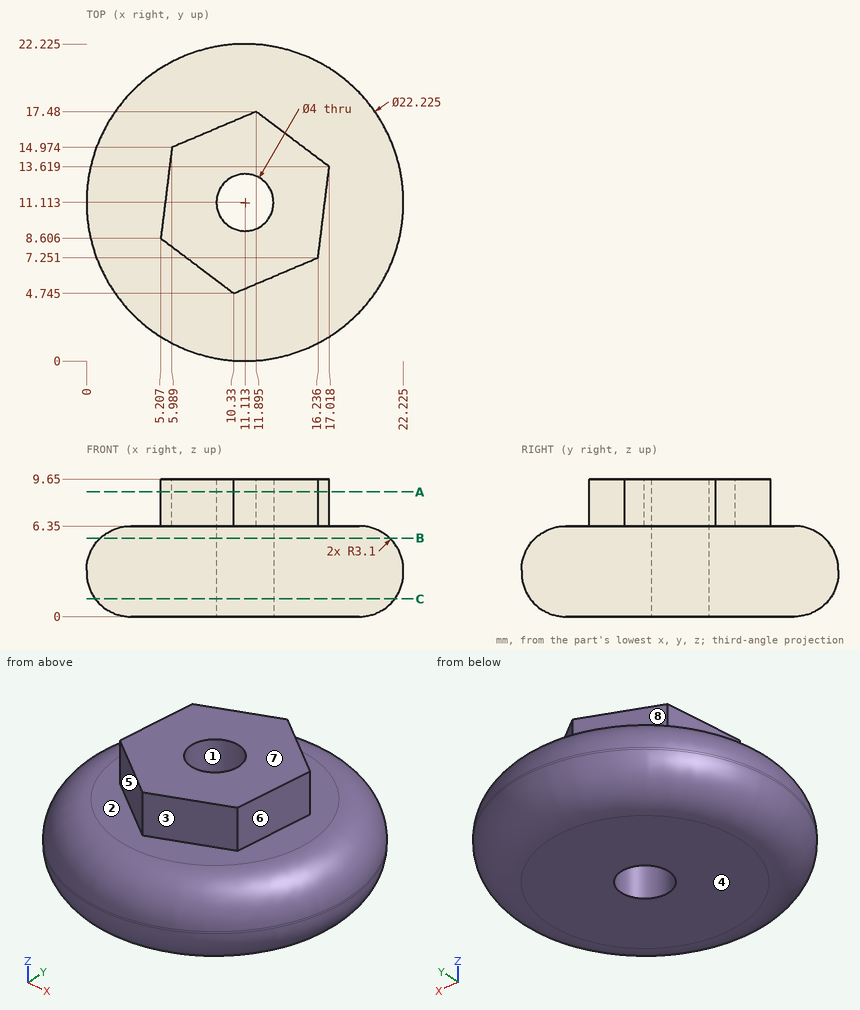
The drawing under review shows one solid part. Ordinate dimensions are in mm from its lowest x, y, z. A direction names the side the tool comes from. Coordinates: 2 decimals unless noted, no trailing zeros. Order: outer loops, then holes, each group sorted by start corner. A loop starts at its lowest first (then second) coordinate and runs counter-clockwise, first axis right, second up. Notation, with made-up numbers: (-24.75, -28) -> (17.25, -28) arc R13 cw to (17.25, -21) -> close; hole circle Ø2 at (8.25, 20.5). An arc over 180 degrees is marked (long way). Answer in a Markdown table with one row per item.
(1) Consider section B-B (z = 5.5). Write out the cut boundary in (x, y) (1 decimal), plus the area to 3 significant figures.
Answers:
| item | result |
|---|---|
| outline | circle Ø20.3 at (11.1, 11.1); hole circle Ø4 at (11.1, 11.1) |
| area | 311 mm² |
(2) The part is to be moulded in two halves that separate along Y. For the marked faces 1, 2 and 3, say which applies: +Y half, -Y half, draft (parallel to the pull), parting line (faces both ways), or undercut.
Answers:
| item | result |
|---|---|
| face 1 | undercut |
| face 2 | draft |
| face 3 | -Y half |
(3) Wall thickness on line 1 along Z through (x, y) = (8, 18.5); line 2 along X through (y, z) = (10.5, 0.5) (1 decimal): over which ranges is each line inside the solid? List them lowest first.
Answers:
| item | result |
|---|---|
| line 1 | 0 to 6.35 |
| line 2 | 1.4 to 9.2, 13 to 20.8 |
(4) Insertion check: pin 1 (5 mm diameter, centred on x = 10, y = 19.5, fed in from +Z); pin 2 (1 mm diameter, centred on y = 16, z = 1.5, fed in from -X) (1 decimal); pin 3 (2 mm diameter, centred on x = 4, y = 4, fed in from -Z). Each pin has a flat end and moves straight along its axis. Give the tip position at first contact, or say it passes through.
Answers:
| item | result |
|---|---|
| pin 1 | z = 6.35 |
| pin 2 | x = 1.3 |
| pin 3 | z = 0.18 |
(5) Consider section A-A (z = 8.75). Write out the cut boundary in (x, y) (1 decimal).
Answers:
| item | result |
|---|---|
| outline | (5.2, 8.6) -> (10.3, 4.7) -> (16.2, 7.3) -> (17, 13.6) -> (11.9, 17.5) -> (6, 15) -> close; hole circle Ø4 at (11.1, 11.1) |
(6) Consider section C-C (z = 1.25). Write out the cut boundary in (x, y), plus the area to 3 significant figures.
Answers:
| item | result |
|---|---|
| outline | circle Ø21 at (11.11, 11.11); hole circle Ø4 at (11.11, 11.11) |
| area | 334 mm² |
(7) Machinability: for the marked faces 4, 5, 6, 7 and 8, which of the approach directions +Z, -Z, +X, -X, +Y, -Y give a long, thin tool a straight path to every point of the face, cutting with its end or side? Answer none if there is none.
Answers:
| item | result |
|---|---|
| face 4 | -Z, +X, -X, +Y, -Y |
| face 5 | +Z, -X, -Y |
| face 6 | +Z, +X, -Y |
| face 7 | +Z, +X, -X, +Y, -Y |
| face 8 | +Z, -X, +Y |
